from build123d import *

# Parameters (mm, degrees)
SCHIZZO1_R                   = 70
ESTRUSIONE_ESTRUSIONE1_DEPTH = 2.2
SCHIZZO2_R                   = 86.5
ESTRUSIONE_ESTRUSIONE2_DEPTH = 140
SCHIZZO3_R                   = 84.3
ESTRUSIONE_ESTRUSIONE3_DEPTH = 2.5
SCHIZZO4_R                   = 81.6
ESTRUSIONE_ESTRUSIONE4_DEPTH = 10.5
SVUOTA1_T                    = -1
RACCORDO1_R                  = 10


with BuildPart() as part:
    # Schizzo1 → Estrusione-Estrusione1 (new body)
    with BuildSketch(Plane.XY):
        Circle(SCHIZZO1_R)
    extrude(amount=ESTRUSIONE_ESTRUSIONE1_DEPTH)

    # Schizzo2 → Estrusione-Estrusione2 (add)
    with BuildSketch(Plane.XY.offset(2.2)):
        Circle(SCHIZZO2_R)
    extrude(amount=ESTRUSIONE_ESTRUSIONE2_DEPTH)

    # Schizzo3 → Estrusione-Estrusione3 (add)
    with BuildSketch(Plane.XY.offset(142.2)):
        Circle(SCHIZZO3_R)
    extrude(amount=ESTRUSIONE_ESTRUSIONE3_DEPTH)

    # Schizzo4 → Estrusione-Estrusione4 (add)
    with BuildSketch(Plane.XY.offset(144.7)):
        with Locations(Location((0, 0, 0), (0, 0, 180))):
            Circle(SCHIZZO4_R)
    extrude(amount=ESTRUSIONE_ESTRUSIONE4_DEPTH)

    # Svuota1
    svuota1_openings = [part.faces().sort_by_distance(p)[0] for p in [
        (0, 0, 155.2),
    ]]
    offset(amount=SVUOTA1_T, openings=svuota1_openings, kind=Kind.INTERSECTION)

    # Raccordo1
    raccordo1_edges = [part.edges().sort_by_distance(p)[0] for p in [
        (-85.5, 0, 3.2),
        (-86.5, 0, 2.2),
    ]]
    fillet(raccordo1_edges, radius=RACCORDO1_R)


solid = part.part
Read the model definition and answer for the solid it produces. Units are mm, in the model's axes. A direction names the side the tool comes from. Round coordinates to 2 decimals unless told otherwise and drop trailing zeros. Write each loop counter-clockwise with the first axis right and the second up, starting at its lowest first coordinate (ties: lowest second). Pieces come first, ordered by that corner, then holes. Notation, with made-up numbers: (21.25, 81.5) - (32.25, 81.5) arc R27 cw to (32.25, 105.5) - close; hole circle Ø8 at (76, -8.5). An arc over 180 degrees is marked (long way). One line per question, with ' | ' between items. Start each with the question number.
1. For faces 5 (the face through (-1, 1, 0)), 6 (the face through (19, -82, 141.2)), 7 (the face through (34, -62, 2.2)), 8 (the face through (33, -61, 3.2)), determine the directions among +Z, -Z, +X, -X, +Y, -Y from which every point of the face is accessible in a straight line to the end or side of a thin tool.
2. Section A-A (z = 98) is taken. Determine the outline of the cut face in (x, y), and give its area (3 significant figures).
3. Each of these flat-tipped pins is pushed along its axis until it touches: pin 1 (5 mm diameter, centred on y = -8, z = 62, fed in from +X); pin 2 (4 mm diameter, centred on x = -67, z = 66.5, fed in from -Y); pin 3 (5 mm diameter, centred on x = 23.5, z = 110, fed in from -Y). Where does it stop, or does it pass through?
4. For a pull along Z with two mould halves and no side action, classify faces 1 (the face through (-68, 44, 143.7)), 2 (the face through (79, -19, 155.2)), 3 (the face through (65.814, 20.726, 2.085)), 4 (the face through (-66.1, -50.69, 142.43)) as +Z half, -Z half, draft (parallel to the pull), parting line (faces both ways), or undercut.
5. Find the intervals of material crossed by probe 1 along Y at (x, z) = (0, 150.25); probe 2 along Z at (x, y) = (16, -32); probe 3 along X at (y, z) = (-56.5, 69), in increasing order. Write a range as [from, to].
Filled in:
1) face 5: -Z, +X, -X, +Y, -Y | face 6: none | face 7: -Z | face 8: +Z
2) outline: circle Ø173 at (0, 0); hole circle Ø171 at (0, 0) | area: 540 mm²
3) pin 1: x = 86.32 | pin 2: y = -57.07 | pin 3: y = -83.91
4) face 1: undercut | face 2: +Z half | face 3: draft | face 4: undercut
5) probe 1: [-81.6, -80.6], [80.6, 81.6] | probe 2: [0, 1] | probe 3: [-65.5, -64.17], [64.17, 65.5]
